Part model, mm, in its own coordinate system. A direction names the side the tool comes from. Round coordinates to 2 decimals unless told otherwise and drop trailing zeros. Loops run counter-clockwise (first coordinate to the right, second up) from the corner with the lowest first, then second, coordinate; pieces in that order, holes last. Notation, with made-up numbers: (79.5, -4.75) -> (91.5, -4.75) arc R22 cw to (91.5, 24.25) -> close; hole circle Ø4 at (87, 50). An arc over 180 degrees is marked (long way). Answer as CSV lines item,"result".
from build123d import *

# Parameters (mm, degrees)
F0_R     = 40
F0_R_2   = 20
F1_DEPTH = 80
F2_W     = 80
F2_H     = 60
F3_DEPTH = 40
F4_R     = 29.99999
F5_DEPTH = 70.001
F6_R     = 10
F7_DEPTH = 80.001


# Not quite as in the source:
# - a fillet or chamfer is up to 0.001 mm smaller than in the source, because OpenCascade refuses the exact size


with BuildPart() as f1:
    # F0 (on Top) → F1 (new body)
    with BuildSketch(Plane.XY):
        Circle(F0_R)
        Circle(F0_R_2, mode=Mode.SUBTRACT)
    extrude(amount=F1_DEPTH)

    # F2 (on Front) → F3 (join, symmetric)
    with BuildSketch(Plane.XZ):
        with Locations((-40, 40)):
            Rectangle(F2_W, F2_H)
    extrude(amount=F3_DEPTH, both=True)

    # F4 (radius 30 in the source; OpenCascade refuses exactly that, so slightly less here)
    f4_edges = [f1.edges().sort_by_distance(p)[0] for p in [
        (-80, 0, 70),
        (-80, 0, 10),
    ]]
    fillet(f4_edges, radius=F4_R)

    # F5 (cut, through all): a face of the model
    f5_faces = [f1.faces().sort_by_distance(p)[0] for p in [
        (-8.4882636316, 0, 70),
    ]]
    extrude(f5_faces, amount=-F5_DEPTH, mode=Mode.SUBTRACT)

    # F6 (on face) → F7 (cut, through all)
    with BuildSketch(Plane.XZ.offset(40)):
        with Locations((-55, 40)):
            Circle(F6_R)
    extrude(amount=-F7_DEPTH, mode=Mode.SUBTRACT)


solid = f1.part
Q1. Drop flat-ended pins along their axis: P1, Ø1, axis at x = -43, y = -30.5, coming from the +Z side; P2, Ø12, axis at x = 12, z = 12, coming from the -Y side; P3, Ø16, axis at x = -55, z = 40, coming from the +Y side; P4, Ø12, axis at x = -59.5, y = 13, coming from the +Z side. Give the stop position or say it passes through.
Geometry results:
P1,"z = 70"
P2,"y = -39.55"
P3,"through"
P4,"z = 69.8"
Q2. Saw through at A-A, the plane y = 0. Give the number of separate pieces and of enclosed holes in the cut face, then the cut area to 3 significant figures.
Geometry results:
separate pieces,"2"
enclosed holes,"1"
area,"4,900 mm2"
Q3. Saw through at B-B, the plane x = -57.5. Write the cut outline in (y, z), then the cut area to 3 significant figures.
Geometry results:
outline,"(-40, 10.95) -> (40, 10.95) -> (40, 30.32) -> (-40, 30.32) -> close; (-40, 49.68) -> (40, 49.68) -> (40, 69.05) -> (-40, 69.05) -> close"
area,"3,100 mm2"
Q4. Saw through at C-C, the plane z = 62.5. Write the cut outline in (x, y), then the cut area to 3 significant figures.
Geometry results:
outline,"(-69.84, -40) -> (0, -40) arc R40 ccw to (0, 40) -> (-69.84, 40) -> close; hole circle Ø40 at (0, 0)"
area,"6,840 mm2"
Q5. Two-plate mould, pull along Y, no slides. Class faces 1 (the face through (-42, -1, 10)), 2 (the face through (-41, -40, 40)), 3 (the face through (-4.336, -19.524, 39.44)), 4 (the face through (-41, 40, 40)): pulls with the +Y half, pulls with the -Y half, needs draft (parallel to the pull), parting line crosses it, or undercut.
Geometry results:
face 1,"needs draft"
face 2,"pulls with the -Y half"
face 3,"undercut"
face 4,"pulls with the +Y half"
Q6. Drill centre lines: line 1 along Y through (x, z) = (0, 39); line 2 along X through (y, z) = (0.5, 31.5); line 3 along Y through (x, z) = (2, 47). Where is each one in solid material? Low to high.
Geometry results:
line 1,"-40 to -20, 20 to 40"
line 2,"-78.77 to -60.27, -49.73 to -19.99, 19.99 to 40"
line 3,"-39.95 to -19.9, 19.9 to 39.95"
Q7. Which spindle directions (+Z, -Z, +X, -X, +Y, -Y) get a long thin tool onto all of the face, cutting with end or side? Do faces 5 (the face through (-42, -1, 70)), 6 (the face through (-71.445, -0.56, 19.021)). Say none if no direction does.
Geometry results:
face 5,"+Z, -X"
face 6,"-Z, -X, +Y, -Y"
